Input: part model. Units: mm. Frame: model coordinates. Face numbers are marked on the shaded views. A direction names the side the tool comes from. Coordinates: 2 decimals unless noted, no trailing zeros. Write each loop counter-clockwise with the first axis right and the second up, starting at its lowest first coordinate (ties: lowest second). Pieces come first, ordered by that corner, then holes.
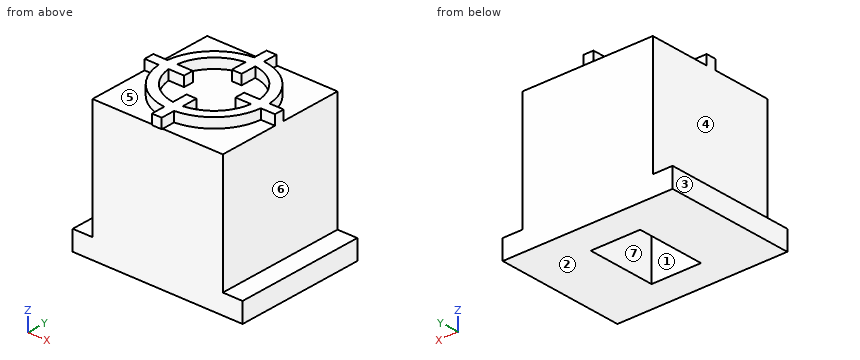
from build123d import *

# Parameters (mm, degrees)
SKETCH040_W      = 0.5
SKETCH040_H      = 2
SKETCH040_W_2    = 2
SKETCH040_H_2    = 0.5
EXTRUDE046_DEPTH = 0.5
SKETCH014_W      = 2.5
SKETCH014_H      = 3.5
EXTRUDE015_DEPTH = 4.5
EXTRUDE014_DEPTH = 6.6
SKETCH038_R      = 2.6
SKETCH038_R_2    = 2.1
EXTRUDE_DEPTH    = 0.5


with BuildPart() as extrude046:
    # Sketch040 → Extrude046 (new body)
    with BuildSketch(Plane.XY.offset(20)):
        with Locations((0, 2.3)):
            Rectangle(SKETCH040_W, SKETCH040_H)
        with Locations((0, -2.3)):
            Rectangle(SKETCH040_W, SKETCH040_H)
        with Locations((-2.3, 0)):
            Rectangle(SKETCH040_W_2, SKETCH040_H_2)
        with Locations((2.3, 0)):
            Rectangle(SKETCH040_W_2, SKETCH040_H_2)
    extrude(amount=EXTRUDE046_DEPTH)


with BuildPart() as extrude046_1:
    # Extrude046 placement: moved
    add(extrude046.part.moved(Location((0, 0, -13))))


with BuildPart() as extrude015:
    # Sketch014 → Extrude015 (new body)
    with BuildSketch(Plane(origin=(0, 0, -10), x_dir=(1, 0, 0), z_dir=(0, 0, -1))):
        Rectangle(SKETCH014_W, SKETCH014_H)
    extrude(amount=-EXTRUDE015_DEPTH)


with BuildPart() as extrude015_1:
    # Extrude015 placement: moved
    add(extrude015.part.moved(Location((0, 0, 10))))


with BuildPart() as cap002:
    # Sketch013 → Extrude014 (new body)
    with BuildSketch(Plane.XZ.offset(10)):
        Polygon((-3.3, 7), (3.3, 7), (3.3, 1), (4.3, 1), (4.3, 0), (-4.3, 0), (-4.3, 1), (-3.3, 1), align=None)
    extrude(amount=-EXTRUDE014_DEPTH)


with BuildPart() as cap002_1:
    # Extrude014 placement: moved
    add(cap002.part.moved(Location((0, 6.75, 0))))

    # Cut023: cut Extrude015
    add(extrude015_1.part, mode=Mode.SUBTRACT)


with BuildPart() as focus:
    # Sketch038 → Extrude (new body)
    with BuildSketch(Plane.XY.offset(20)):
        Circle(SKETCH038_R)
        Circle(SKETCH038_R_2, mode=Mode.SUBTRACT)
    extrude(amount=EXTRUDE_DEPTH)


with BuildPart() as focus_1:
    # Extrude placement: moved
    add(focus.part.moved(Location((0, 0, -13))))

    # Fusion034: union Extrude046, cap002
    add(extrude046_1.part)
    add(cap002_1.part)


with BuildPart() as focus_2:
    # Fusion034 placement: moved
    add(focus_1.part.moved(Location((2, 0, 50))))


solid = focus_2.part
Item 1: Section query D-D, the plane z = 54. Return loops of the section in (x, y).
Item 2: Material intervals for line 1 (X direction, y = 0.25, z = 53.25); line 2 (Z direction, x = 5, y = 2.75); line 3 (X direction, y = 1.25, z = 50.75), sorted ascending.
Item 3: Pin query (flat end, axial travel): pin 1 Ø4 at (x, z) = (-1, 51.5) entering from -Y; pin 2 Ø0.6 at (y, z) = (1.5, 57) entering from +X; pin 3 Ø0.9 at (x, y) = (4.5, -2.5) entering from +Z. Return the tip coordinate at first contact, or that it passes through.
Item 4: Access query for the marked faces 4, 5, 6 and 7. Directions: +Z, -Z, +X, -X, +Y, -Y. A direction counts if a zero-diameter tool reaches every point of the face in a straight line with its end or side. Return the directions, or none.
Item 5: Pull-direction query (X, two-part tool) for the marked faces 1, 2 and 3; classes: released by +X, released by -X, zero draft, split by the parting line, or undercut.
Item 6: Section query C-C, the plane x = -1. Return loops of the section in (y, z), then the cut area to 4 significant figures.
Item 7: Section query B-B, the plane y = 3. Return loops of the section in (x, z).
The answers:
1. outline: (-1.3, -3.25) - (5.3, -3.25) - (5.3, 3.35) - (-1.3, 3.35) - close; hole (0.75, -1.75) - (3.25, -1.75) - (3.25, 1.75) - (0.75, 1.75) - close
2. line 1: x = -1.3 to 0.75, 3.25 to 5.3
2. line 2: z = 50 to 57
2. line 3: x = -2.3 to 0.75, 3.25 to 6.3
3. pin 1: stops at y = -3.25
3. pin 2: stops at x = 5.3
3. pin 3: stops at z = 57
4. face 4: +Z, -X, +Y, -Y
4. face 5: +Z, -X, -Y
4. face 6: +Z, +X, +Y, -Y
4. face 7: -Z
5. face 1: undercut
5. face 2: zero draft
5. face 3: released by -X
6. outline: (-3.25, 50) - (3.35, 50) - (3.35, 57) - (0.25, 57) - (0.25, 57.5) - (-0.25, 57.5) - (-0.25, 57) - (-3.25, 57) - close
6. area: 46.45 mm2
7. outline: (-2.3, 50) - (6.3, 50) - (6.3, 51) - (5.3, 51) - (5.3, 57) - (2.25, 57) - (2.25, 57.5) - (1.75, 57.5) - (1.75, 57) - (-1.3, 57) - (-1.3, 51) - (-2.3, 51) - close
